Check sheet for the modelled part. Datum: model origin and axes. Units: mm. A direction names the side the tool comes from. Coordinates: 2 decimals unless noted, no trailing zeros. Loops run counter-clockwise (first coordinate to the right, second up) from the corner with the lowest first, then second, coordinate; pieces in that order, holes last. Notation, with made-up numbers: (3.25, 56.25) - (53.25, 56.25) arc R31 ccw to (53.25, 87.25) - close; hole circle Ø4 at (70.25, -35.5). An arc over 180 degrees is marked (long way). Write each question's results on one line, items separated by ' | '. Start each with the question number.
1. Cross-section at A-A (x = 10). Record the cut outline in (y, z), and give its area (3 significant figures).
2. Cross-section at B-B (y = 71). Record the cut outline in (x, z), and give its area (3 significant figures).
3. Draft check along X on faces 1 (the face through (1, 38.5, 18)), 2 (the face through (77, 2, 42)), 3 (the face through (155, 54, 39)). Enter one of: released by +X, released by -X, zero draft, split by the parting line, or undercut.
4. Gauge pin test, flat ends, axial feed: P1, Ø4.5, axis at x = 10, y = 100.5, coming from the -Z side; P2, Ø2, axis at x = 154, y = 83.5, coming from the -Z side; P3, Ø1.5, axis at x = 136.5, y = 44, coming from the +Z side; P4, Ø4, axis at y = 58.5, z = 53, coming from the -X side. Record the tip position at first contact, or that the pin passes through.
5. Tool access check on faces 4 (the face through (153, 54, 33)), 5 (the face through (1, 55.1, 17.5)), 6 (the face through (43.21, 109.01, 21.12)). Record the directions out of +Z, -Z, +X, -X, +Y, -Y that give a thin tool (end or side, any length) a straight path to the whole face; none if there is none.
6. Thickness scan on line 1 (Z direction, x = 0.95, y = 92.5); line 2 (Y direction, x = 14, z = 51.5); line 3 (Z direction, x = 95.28, y = 108.6). Record the ranges inside material, lowest first. Write a range as [from, to].
7. Cross-section at C-C (x = 139). Record the cut outline in (y, z).
```python
from build123d import *

# Parameters (mm, degrees)
SKETCH1_W           = 155
SKETCH1_H           = 110
BOSS_EXTRUDE1_DEPTH = 80
SKETCH2_W           = 151
SKETCH2_H           = 106
CUT_EXTRUDE1_DEPTH  = 78
SKETCH3_R           = 2.5
CUT_EXTRUDE2_DEPTH  = 2
SKETCH7_R           = 1.6
CUT_EXTRUDE7_DEPTH  = 2
SKETCH4_W           = 27.5
SKETCH4_H           = 46.8
CUT_EXTRUDE8_DEPTH  = 2
SKETCH8_W           = 4
SKETCH8_H           = 53
CUT_EXTRUDE9_DEPTH  = 2
SKETCH9_W           = 14
SKETCH9_H           = 14
CUT_EXTRUDE10_DEPTH = 2
SKETCH10_W          = 25.2
SKETCH10_H          = 71.2
SKETCH10_R          = 1.25
CUT_EXTRUDE12_DEPTH = 2
SKETCH11_R          = 2.5
SKETCH11_R_2        = 4.5
CUT_EXTRUDE13_DEPTH = 2


with BuildPart() as part:
    # Sketch1 → Boss-Extrude1 (new body)
    with BuildSketch(Plane.XY):
        with Locations((77.5, 55)):
            Rectangle(SKETCH1_W, SKETCH1_H)
    extrude(amount=BOSS_EXTRUDE1_DEPTH)

    # Sketch2 → Cut-Extrude1 (cut)
    with BuildSketch(Plane.XY.offset(80)):
        with Locations((77.5, 55)):
            Rectangle(SKETCH2_W, SKETCH2_H)
    extrude(amount=-CUT_EXTRUDE1_DEPTH, mode=Mode.SUBTRACT)

    # Sketch3 → Cut-Extrude2 (cut)
    with BuildSketch(Plane.XY.offset(2)):
        with Locations((145, 100.5)):
            Circle(SKETCH3_R)
        with Locations((145, 9.5)):
            Circle(SKETCH3_R)
        with Locations((10, 9.5)):
            Circle(SKETCH3_R)
        with Locations((10, 100.5)):
            Circle(SKETCH3_R)
    extrude(amount=-CUT_EXTRUDE2_DEPTH, mode=Mode.SUBTRACT)

    # Sketch7 → Cut-Extrude7 (cut)
    with BuildSketch(Plane(origin=(0, 110, 0), x_dir=(1, 0, 0), z_dir=(0, 1, 0))):
        with Locations((44.48, -20.14450396)):
            Circle(SKETCH7_R)
        with Locations((95.28, -17.14)):
            Circle(SKETCH7_R)
        with Locations((95.28, -62.86)):
            Circle(SKETCH7_R)
        with Locations((44.48, -47.62)):
            Circle(SKETCH7_R)
    extrude(amount=-CUT_EXTRUDE7_DEPTH, mode=Mode.SUBTRACT)

    # Sketch4 → Cut-Extrude8 (cut)
    with BuildSketch(Plane(origin=(155, 0, 0), x_dir=(0, 0, -1), z_dir=(1, 0, 0))):
        with Locations((-40, 82.5)):
            Rectangle(SKETCH4_W, SKETCH4_H)
    extrude(amount=-CUT_EXTRUDE8_DEPTH, mode=Mode.SUBTRACT)

    # Sketch8 → Cut-Extrude9 (cut)
    with BuildSketch(Plane(origin=(155, 0, 0), x_dir=(0, 0, -1), z_dir=(1, 0, 0))):
        with Locations((-68, 28.5)):
            Rectangle(SKETCH8_W, SKETCH8_H)
        with Locations((-76, 28.5)):
            Rectangle(SKETCH8_W, SKETCH8_H)
        with Locations((-60, 28.5)):
            Rectangle(SKETCH8_W, SKETCH8_H)
        with Locations((-52, 28.5)):
            Rectangle(SKETCH8_W, SKETCH8_H)
        with Locations((-44, 28.5)):
            Rectangle(SKETCH8_W, SKETCH8_H)
        with Locations((-36, 28.5)):
            Rectangle(SKETCH8_W, SKETCH8_H)
        with Locations((-28, 28.5)):
            Rectangle(SKETCH8_W, SKETCH8_H)
        with Locations((-20, 28.5)):
            Rectangle(SKETCH8_W, SKETCH8_H)
        with Locations((-12, 28.5)):
            Rectangle(SKETCH8_W, SKETCH8_H)
        with Locations((-4, 28.5)):
            Rectangle(SKETCH8_W, SKETCH8_H)
    extrude(amount=-CUT_EXTRUDE9_DEPTH, mode=Mode.SUBTRACT)

    # Sketch9 → Cut-Extrude10 (cut)
    with BuildSketch(Plane(origin=(0, 110, 0), x_dir=(1, 0, 0), z_dir=(0, 1, 0))):
        with Locations((120, -19)):
            Rectangle(SKETCH9_W, SKETCH9_H)
    extrude(amount=-CUT_EXTRUDE10_DEPTH, mode=Mode.SUBTRACT)

    # Sketch10 → Cut-Extrude12 (cut)
    with BuildSketch(Plane.ZY):
        with Locations((58, 55)):
            Rectangle(SKETCH10_W, SKETCH10_H)
        with Locations((42.5, 92.5)):
            Circle(SKETCH10_R)
        with Locations((73.5, 92.5)):
            Circle(SKETCH10_R)
        with Locations((42.5, 17.5)):
            Circle(SKETCH10_R)
        with Locations((73.5, 17.5)):
            Circle(SKETCH10_R)
    extrude(amount=-CUT_EXTRUDE12_DEPTH, mode=Mode.SUBTRACT)

    # Sketch11 → Cut-Extrude13 (cut)
    with BuildSketch(Plane.ZY):
        with Locations((20, 55)):
            Circle(SKETCH11_R)
        with Locations((20, 40)):
            Circle(SKETCH11_R)
        with Locations((20, 25)):
            Circle(SKETCH11_R)
        with Locations((20, 82.5)):
            Circle(SKETCH11_R_2)
    extrude(amount=-CUT_EXTRUDE13_DEPTH, mode=Mode.SUBTRACT)


solid = part.part
```
Established:
1) outline: (0, 0) - (7, 0) - (7, 2) - (2, 2) - (2, 80) - (0, 80) - close; (12, 0) - (98, 0) - (98, 2) - (12, 2) - close; (103, 0) - (110, 0) - (110, 80) - (108, 80) - (108, 2) - (103, 2) - close | area: 512 mm^2
2) outline: (0, 0) - (155, 0) - (155, 26.25) - (153, 26.25) - (153, 2) - (2, 2) - (2, 45.4) - (0, 45.4) - close; (0, 70.6) - (2, 70.6) - (2, 80) - (0, 80) - close; (153, 53.75) - (155, 53.75) - (155, 80) - (153, 80) - close | area: 517 mm^2
3) face 1: zero draft | face 2: undercut | face 3: released by +X
4) P1: through | P2: z = 0 | P3: z = 2 | P4: x = 153
5) face 4: +Z | face 5: -X | face 6: +Y
6) line 1: [0, 41.25], [43.75, 72.25], [74.75, 80] | line 2: [0, 2], [108, 110] | line 3: [0, 15.54], [18.74, 61.26], [64.46, 80]
7) outline: (0, 0) - (110, 0) - (110, 80) - (108, 80) - (108, 2) - (2, 2) - (2, 80) - (0, 80) - close
